Work out the finished part from the listing and answer in its coordinate system (mm). A direction names the side the tool comes from. Give positions to 0.01 mm unless a question says otherwise; leave off trailing zeros. Loops run counter-clockwise (first coordinate to the right, second up) from the corner with the lowest first, then second, coordinate; pieces in that order, holes last. Notation, with made-up numbers: (17, 3.25) - (48, 3.25) arc R16 ccw to (48, 34.25) - close; hole circle Ø4 at (29, -27). An arc over 180 degrees is marked (long way). One line per question, with ' | ' between items. Start each with the question number.
1. Section C-C (y = 7.75) is taken. Determine the outline of the cut face in (x, z).
2. For a pull along Z with two mould halves and no side action, classify faces 5 (the face through (18.5, 55.2, -60.3)), 6 (the face through (11, -2, -36.5)) as released by +Z, released by -Z, zero draft, split by the parting line, or undercut.
3. Section D-D (z = -67.55) is taken. Determine the outline of the cut face in (x, y).
4. Each of these flat-tipped pins is pushed along its axis until it touches: pin 1 (1.6 mm diameter, centred on x = 4.5, y = 12, fed in from -Z); pin 2 (4 mm diameter, centred on y = 57.5, z = -4, fed in from -X); pin 3 (0.7 mm diameter, centred on y = 54, z = -4, fed in from +X). Where does it stop, or does it pass through?
5. Find the intervals of material crossed by line 1 (Y direction, x = 0.95, z = -14.25); line 2 (Z direction, x = 6, y = 23.5); line 3 (Y direction, x = 1.2, z = -67.55), in increasing order.
6. Section B-B (y = 41.25) is taken. Determine the outline of the cut face in (x, z), plus the area to 3 significant figures.
7. Which of the six approach directions +Z, -Z, +X, -X, +Y, -Y give full straight-line access (tool end or side, diameter ignored) to faces 1 (the face through (5, 1, -42.2)), 2 (the face through (6, 57, -38)), 3 (the face through (12, 20.75, 2)), 4 (the face through (2, 56, -7.9))?
8. Section A-A (z = -55) is taken. Determine the outline of the cut face in (x, y).
from build123d import *

# Parameters (mm, degrees)
SKETCH_1_W          = 88
SKETCH_1_H          = 62
EXTRUDE_1_DEPTH     = 3.5
SKETCH_2_W          = 88
SKETCH_2_H          = 62
SKETCH_2_W_2        = 81
SKETCH_2_H_2        = 55
EXTRUDE_2_DEPTH     = 15
SKETCH_3_R          = 2.5
EXTRUDE_3_DEPTH     = 4
SKETCH_4_W          = 3
SKETCH_4_H          = 34
SKETCH_4_W_2        = 2.683429954
SKETCH_4_H_2        = 10.857152268
CUT_EXTRUDE_2_DEPTH = 3.5
SKETCH_7_W          = 8.5
SKETCH_7_H          = 11
SKETCH_7_H_2        = 13
SKETCH_7_W_2        = 7.5
SKETCH_7_H_3        = 2.5
CUT_EXTRUDE_3_DEPTH = 4
SKETCH_8_W          = 12
SKETCH_8_H          = 8
CUT_EXTRUDE_4_DEPTH = 3.5
CUT_EXTRUDE_5_DEPTH = 3.5
SKETCH_10_R         = 1.7
CUT_EXTRUDE_6_DEPTH = 3.5
EXTRUDE_4_DEPTH     = 3
SKETCH_12_W         = 6
SKETCH_12_H         = 5.75
SKETCH_12_W_2       = 5.75
SKETCH_12_H_2       = 6
CUT_EXTRUDE_7_DEPTH = 3.25
SKETCH_13_W         = 29
SKETCH_13_H         = 3.5
EXTRUDE_5_DEPTH     = 2


with BuildPart() as part:
    # 草图1 → 凸台-拉伸1 (new body)
    with BuildSketch(Plane(origin=(0, 0, 0), x_dir=(0, 0, -1), z_dir=(1, 0, 0))):
        with Locations((40.5, 27.5)):
            Rectangle(SKETCH_1_W, SKETCH_1_H)
    extrude(amount=EXTRUDE_1_DEPTH)

    # 草图2 → 凸台-拉伸2 (add)
    with BuildSketch(Plane(origin=(3.5, 0, 0), x_dir=(0, 0, -1), z_dir=(1, 0, 0))):
        with Locations((40.5, 27.5)):
            Rectangle(SKETCH_2_W, SKETCH_2_H)
        with Locations((40.5, 27.5)):
            Rectangle(SKETCH_2_W_2, SKETCH_2_H_2, mode=Mode.SUBTRACT)
    extrude(amount=EXTRUDE_2_DEPTH)

    # 草图3 → 凸台-拉伸3 (add)
    with BuildSketch(Plane(origin=(3.5, 0, 0), x_dir=(0, 0, -1), z_dir=(1, 0, 0))):
        with Locations((20.25, 41.25)):
            Circle(SKETCH_3_R)
        with Locations((60.75, 41.25)):
            Circle(SKETCH_3_R)
        with Locations((60.75, 13.75)):
            Circle(SKETCH_3_R)
        with Locations((20.25, 13.75)):
            Circle(SKETCH_3_R)
    extrude(amount=EXTRUDE_3_DEPTH)

    # 草图4 → 切除-拉伸2 (cut)
    with BuildSketch(Plane(origin=(0, 58.5, 0), x_dir=(1, 0, 0), z_dir=(0, 1, 0))):
        with Locations((6, 55)):
            Rectangle(SKETCH_4_W, SKETCH_4_H)
        Polygon((7.5, 38), (6.816570046, 38), (6.816570046, 9), (15.816570046, 9), (15.816570046, 11.869210194), (15.816570046, 22.726362462), (15.816570046, 38), align=None)
        Polygon((0, 3.2), (7.5, 3.2), (7.5, 2.2), (15.5, 2.2), (15.5, 7.6), (7.5, 7.6), (7.5, 6.6), (0, 6.6), align=None)
        with Locations((17.158285023, 17.297786328)):
            Rectangle(SKETCH_4_W_2, SKETCH_4_H_2)
    extrude(amount=-CUT_EXTRUDE_2_DEPTH, mode=Mode.SUBTRACT)

    # 草图7 → 切除-拉伸3 (cut)
    with BuildSketch(Plane.XY.offset(3.5)):
        with Locations((11.75, 26.25)):
            Rectangle(SKETCH_7_W, SKETCH_7_H)
        with Locations((11.75, 42.5)):
            Rectangle(SKETCH_7_W, SKETCH_7_H_2)
        with Locations((3.75, 27.5)):
            Rectangle(SKETCH_7_W_2, SKETCH_7_H_3)
        with Locations((3.75, 25)):
            Rectangle(SKETCH_7_W_2, SKETCH_7_H_3)
    extrude(amount=-CUT_EXTRUDE_3_DEPTH, mode=Mode.SUBTRACT)

    # 草图8 → 切除-拉伸4 (cut)
    with BuildSketch(Plane.XZ.offset(3.5)):
        with Locations((13.5, -19)):
            Rectangle(SKETCH_8_W, SKETCH_8_H)
        Polygon((7.5, -36.5), (15.5, -36.5), (15.5, -41.9), (7.5, -41.9), (7.5, -40.9), (0, -40.9), (0, -37.5), (7.5, -37.5), align=None)
    extrude(amount=-CUT_EXTRUDE_4_DEPTH, mode=Mode.SUBTRACT)

    # 草图9 → 切除-拉伸5 (cut)
    with BuildSketch(Plane(origin=(0, 0, -84.5), x_dir=(-1, 0, 0), z_dir=(0, 0, -1))):
        Polygon((-7.5, 11), (0, 11), (0, 14.4), (-7.5, 14.4), (-7.5, 15.4), (-15.5, 15.4), (-15.5, 10), (-7.5, 10), align=None)
    extrude(amount=-CUT_EXTRUDE_5_DEPTH, mode=Mode.SUBTRACT)

    # 草图10 → 切除-拉伸6 (cut)
    with BuildSketch(Plane(origin=(3.5, 0, 0), x_dir=(0, 0, -1), z_dir=(1, 0, 0))):
        with Locations((14.25, 47.25)):
            Circle(SKETCH_10_R)
        with Locations((14.25, 7.75)):
            Circle(SKETCH_10_R)
        with Locations((67.55, 7.75)):
            Circle(SKETCH_10_R)
    extrude(amount=-CUT_EXTRUDE_6_DEPTH, mode=Mode.SUBTRACT)

    # 草图11 → 凸台-拉伸4 (add)
    with BuildSketch(Plane(origin=(3.5, 0, 0), x_dir=(0, 0, -1), z_dir=(1, 0, 0))):
        Polygon((40.9, 0), (42.2, 0), (42.2, 2.25), (36.2, 2.25), (36.2, 0), (37.5, 0), align=None)
        Polygon((81, 14.4), (81, 15.7), (78.75, 15.7), (78.75, 9.7), (81, 9.7), (81, 11), align=None)
        Polygon((4.9, 52.75), (4.9, 55), (3.2, 55), (1.9, 55), (1.9, 52.75), align=None)
        Polygon((6.6, 55), (4.9, 55), (4.9, 52.75), (7.9, 52.75), (7.9, 55), align=None)
    extrude(amount=EXTRUDE_4_DEPTH)

    # 草图12 → 切除-拉伸7 (cut)
    with BuildSketch(Plane.ZY):
        with Locations((-4.9, 55.625)):
            Rectangle(SKETCH_12_W, SKETCH_12_H)
        with Locations((-39.2, -0.625)):
            Rectangle(SKETCH_12_W, SKETCH_12_H)
        with Locations((-81.625, 12.7)):
            Rectangle(SKETCH_12_W_2, SKETCH_12_H_2)
    extrude(amount=-CUT_EXTRUDE_7_DEPTH, mode=Mode.SUBTRACT)

    # 草图13 → 凸台-拉伸5 (add)
    with BuildSketch(Plane(origin=(6.816570046, 0, 0), x_dir=(0, 0, -1), z_dir=(1, 0, 0))):
        with Locations((23.5, 56.75)):
            Rectangle(SKETCH_13_W, SKETCH_13_H)
    extrude(amount=EXTRUDE_5_DEPTH)


solid = part.part
Conclusion:
1) outline: (0, -84.5) - (18.5, -84.5) - (18.5, -81) - (3.5, -81) - (3.5, -69.25) - (0, -69.25) - close; (0, -65.85) - (3.5, -65.85) - (3.5, -15.95) - (0, -15.95) - close; (0, -12.55) - (3.5, -12.55) - (3.5, 0) - (18.5, 0) - (18.5, 3.5) - (0, 3.5) - close
2) face 5: zero draft | face 6: undercut
3) outline: (0, -3.5) - (18.5, -3.5) - (18.5, 0) - (3.5, 0) - (3.5, 6.05) - (0, 6.05) - close; (0, 9.45) - (3.5, 9.45) - (3.5, 55) - (4.5, 55) - (4.5, 58.5) - (0, 58.5) - close; (7.5, 55) - (18.5, 55) - (18.5, 58.5) - (7.5, 58.5) - close
4) pin 1: z = -81 | pin 2: x = 3.25 | pin 3: x = 6.5
5) line 1: -3.5 to 6.05, 9.45 to 45.55, 48.95 to 58.5 | line 2: -84.5 to -81, 0 to 3.5 | line 3: -3.5 to 6.05, 9.45 to 58.5
6) outline: (0, -84.5) - (18.5, -84.5) - (18.5, -81) - (3.5, -81) - (3.5, -63.25) - (7.5, -63.25) - (7.5, -58.25) - (3.5, -58.25) - (3.5, -22.75) - (7.5, -22.75) - (7.5, -17.75) - (3.5, -17.75) - (3.5, 0) - (7.5, 0) - (7.5, 3.5) - (0, 3.5) - close; (16, 0) - (18.5, 0) - (18.5, 3.5) - (16, 3.5) - close | area: 423 mm²
7) face 1: +X | face 2: +Y | face 3: +Z | face 4: -X, +Y
8) outline: (0, -3.5) - (18.5, -3.5) - (18.5, 0) - (3.5, 0) - (3.5, 55) - (4.5, 55) - (4.5, 58.5) - (0, 58.5) - close; (7.5, 55) - (18.5, 55) - (18.5, 58.5) - (7.5, 58.5) - close
